from build123d import *

# Parameters (mm, degrees)
BOSS_EXTRUDE1_DEPTH = 4
CUT_EXTRUDE1_DEPTH  = 10


with BuildPart() as part:
    # Sketch1 → Boss-Extrude1 (new body)
    with BuildSketch(Plane(origin=(0, 0, 0), x_dir=(1, 0, 0), z_dir=(0, 1, 0))):
        Polygon((-17.714285714, 14), (-17.714285714, 12), (-21.714285714, 12), (-21.714285714, 8), (-17.714285714, 8), (-17.714285714, -4), (-21.714285714, -4), (-21.714285714, -8), (-17.714285714, -8), (-17.714285714, -20), (-21.714285714, -20), (-21.714285714, -24), (-17.714285714, -24), (-17.714285714, -36), (-21.714285714, -36), (-21.714285714, -40), (-17.714285714, -40), (-17.714285714, -52), (-21.714285714, -52), (-21.714285714, -56), (-17.714285714, -56), (-17.714285714, -58), (78.285714286, -58), (78.285714286, -48), (82.285714286, -48), (82.285714286, -44), (78.285714286, -44), (78.285714286, -32), (82.285714286, -32), (82.285714286, -28), (78.285714286, -28), (78.285714286, -16), (82.285714286, -16), (82.285714286, -12), (78.285714286, -12), (78.285714286, 0), (82.285714286, 0), (82.285714286, 4), (78.285714286, 4), (78.285714286, 14), align=None)
    extrude(amount=-BOSS_EXTRUDE1_DEPTH)

    # Sketch2 → Cut-Extrude1 (cut)
    with BuildSketch(Plane(origin=(0, 0, 0), x_dir=(1, 0, 0), z_dir=(0, 1, 0))):
        with BuildLine():
            Line((-4.859302854, 10), (25.285714286, 10))
            ThreePointArc((25.285714286, 10), (26.699927848, 9.414213562), (27.285714286, 8))
            Line((27.285714286, 8), (27.285714286, -11.94278394))
            ThreePointArc((27.285714286, -11.94278394), (26.23255212, -13.704458744), (24.182216171, -13.610804297))
            Line((24.182216171, -13.610804297), (-5.962800969, 6.331979643))
            ThreePointArc((-5.962800969, 6.331979643), (-6.774510508, 8.576176746), (-4.859302854, 10))
        make_face()
        with BuildLine():
            Line((33.285714286, 8), (33.285714286, -11.94278394))
            ThreePointArc((33.285714286, -11.94278394), (34.338876451, -13.704458744), (36.3892124, -13.610804297))
            Line((36.3892124, -13.610804297), (66.53422954, 6.331979643))
            ThreePointArc((66.53422954, 6.331979643), (67.345939079, 8.576176746), (65.430731426, 10))
            Line((65.430731426, 10), (35.285714286, 10))
            ThreePointArc((35.285714286, 10), (33.871500723, 9.414213562), (33.285714286, 8))
        make_face()
        with BuildLine():
            ThreePointArc((74.285714286, -17), (73.699927848, -18.414213562), (72.285714286, -19))
            Line((72.285714286, -19), (42.140697146, -19))
            ThreePointArc((42.140697146, -19), (40.225489492, -17.576176746), (41.037199031, -15.331979643))
            Line((41.037199031, -15.331979643), (71.182216171, 4.610804297))
            ThreePointArc((71.182216171, 4.610804297), (73.23255212, 4.704458744), (74.285714286, 2.94278394))
            Line((74.285714286, 2.94278394), (74.285714286, -17))
        make_face()
        with BuildLine():
            ThreePointArc((74.285714286, -46.94278394), (73.23255212, -48.704458744), (71.182216171, -48.610804297))
            Line((71.182216171, -48.610804297), (41.037199031, -28.668020357))
            ThreePointArc((41.037199031, -28.668020357), (40.225489492, -26.423823254), (42.140697146, -25))
            Line((42.140697146, -25), (72.285714286, -25))
            ThreePointArc((72.285714286, -25), (73.699927848, -25.585786438), (74.285714286, -27))
            Line((74.285714286, -27), (74.285714286, -46.94278394))
        make_face()
        with BuildLine():
            Line((65.430731426, -54), (35.285714286, -54))
            ThreePointArc((35.285714286, -54), (33.871500723, -53.414213562), (33.285714286, -52))
            Line((33.285714286, -52), (33.285714286, -32.05721606))
            ThreePointArc((33.285714286, -32.05721606), (34.338876451, -30.295541256), (36.3892124, -30.389195703))
            Line((36.3892124, -30.389195703), (66.53422954, -50.331979643))
            ThreePointArc((66.53422954, -50.331979643), (67.345939079, -52.576176746), (65.430731426, -54))
        make_face()
        with BuildLine():
            Line((27.285714286, -52), (27.285714286, -32.05721606))
            ThreePointArc((27.285714286, -32.05721606), (26.23255212, -30.295541256), (24.182216171, -30.389195703))
            Line((24.182216171, -30.389195703), (-5.962800969, -50.331979643))
            ThreePointArc((-5.962800969, -50.331979643), (-6.774510508, -52.576176746), (-4.859302854, -54))
            Line((-4.859302854, -54), (25.285714286, -54))
            ThreePointArc((25.285714286, -54), (26.699927848, -53.414213562), (27.285714286, -52))
        make_face()
        with BuildLine():
            ThreePointArc((-13.714285714, -27), (-13.128499277, -25.585786438), (-11.714285714, -25))
            Line((-11.714285714, -25), (18.430731426, -25))
            ThreePointArc((18.430731426, -25), (20.345939079, -26.423823254), (19.53422954, -28.668020357))
            Line((19.53422954, -28.668020357), (-10.6107876, -48.610804297))
            ThreePointArc((-10.6107876, -48.610804297), (-12.661123549, -48.704458744), (-13.714285714, -46.94278394))
            Line((-13.714285714, -46.94278394), (-13.714285714, -27))
        make_face()
        with BuildLine():
            ThreePointArc((-13.714285714, 2.94278394), (-12.661123549, 4.704458744), (-10.6107876, 4.610804297))
            Line((-10.6107876, 4.610804297), (19.53422954, -15.331979643))
            ThreePointArc((19.53422954, -15.331979643), (20.345939079, -17.576176746), (18.430731426, -19))
            Line((18.430731426, -19), (-11.714285714, -19))
            ThreePointArc((-11.714285714, -19), (-13.128499277, -18.414213562), (-13.714285714, -17))
            Line((-13.714285714, -17), (-13.714285714, 2.94278394))
        make_face()
    extrude(amount=-CUT_EXTRUDE1_DEPTH, mode=Mode.SUBTRACT)


solid = part.part
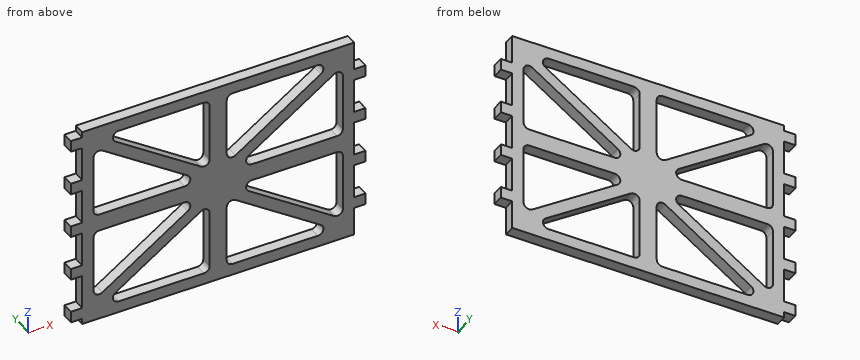
Input: part model. Units: mm. Frame: model coordinates. Give positions to 0.01 mm unless a question says otherwise; leave off trailing zeros. Write each loop counter-clockwise with the first axis right and the second up, starting at its lowest first coordinate (ties: lowest second). Pieces come first, ordered by that corner, then holes. Notation, with made-up numbers: M 3.25,65 L 41.25,65 A21 cw 41.25,77 Z; hole C 37.25,18 d5. An arc over 180 degrees is marked long. Write item = value, one per line. Start each with the question number.
1) Cut plane A-A on x = 56. Return the cut outline in (y, z), then the cut area to 3 significant figures.
2) Cut plane C-C on x = 69. Return the cut outline in (y, z), then the cut area to 3 significant figures.
3) Cut plane B-B on z = 34.5. Return the cut outline in (x, y).
4) Cut plane D-D on y = -2.1. Count the separate pieces of the cut face and the enclosed holes in it, then the cut area to 3 significant figures.
5) Material intervals for line 1 along Z through (x, y) = (72.5, -2.5); line 2 along Z through (x, y) = (-13, -0.2); line 3 along X through (y, z) = (-3, 13), sorted ascending. Write a range as [from, to].
6) First-contact query: pin 1 Ø1.2 at (y, z) = (-1.5, 2) entering from -X; pin 2 Ø12 at (x, z) = (69.5, 23) entering from +Y; pin 3 Ø1.2 at (x, y) = (80.5, -2) entering from +Z; pin 4 Ø2 at (x, y) = (79.5, -2.5) entering from -Z. Flat tips, straight axial feed; report the tip coordinate or a pass-through.
Solved:
q1.outline = M -4,-14 L 0,-14 L 0,-10 L -4,-10 Z; M -4,0.64 L 0,0.64 L 0,5.43 L -4,5.43 Z; M -4,19 L 0,19 L 0,25 L -4,25 Z; M -4,38.57 L 0,38.57 L 0,43.36 L -4,43.36 Z; M -4,54 L 0,54 L 0,58 L -4,58 Z
q1.area = 94.4 mm2
q2.outline = M -4,-14 L 0,-14 L 0,-3.17 L -4,-3.17 Z; M -4,19 L 0,19 L 0,25 L -4,25 Z; M -4,47.17 L 0,47.17 L 0,58 L -4,58 Z
q2.area = 111 mm2
q3.outline = M -17.71,-4 L -13.71,-4 L -13.71,0 L -17.71,0 Z; M 10.72,-4 L 17.97,-4 L 17.97,0 L 10.72,0 Z; M 27.29,-4 L 33.29,-4 L 33.29,0 L 27.29,0 Z; M 42.6,-4 L 49.85,-4 L 49.85,0 L 42.6,0 Z; M 74.29,-4 L 78.29,-4 L 78.29,0 L 74.29,0 Z
q4.separate_pieces = 1
q4.enclosed_holes = 8
q4.area = 3,170 mm2
q5.line_1 = [-14, -4.93], [18.99, 25.01], [48.93, 58]
q5.line_2 = [-14, -4.47], [18.53, 25.47], [48.47, 58]
q5.line_3 = [-17.71, -13.71], [16.01, 23.26], [26.98, 33.59], [37.31, 44.56], [74.29, 82.29]
q6.pin_1 = -17.71
q6.pin_2 = 0
q6.pin_3 = 48
q6.pin_4 = -4
